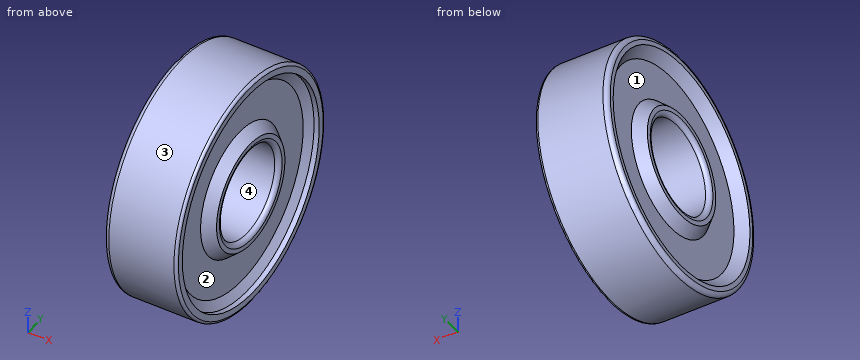
```python
from build123d import *


with BuildPart() as part:
    # Эскиз1 → Повернуть1 (revolve)
    with BuildSketch(Plane.XY):
        with BuildLine():
            Line((-3.5, 13), (3.7, 13))
            ThreePointArc((3.7, 13), (3.912132034, 12.912132034), (4, 12.7))
            Line((4, 12.7), (4, 12))
            Line((4, 12), (3.434493126, 12))
            Line((3.434493126, 12), (2.857142857, 11))
            Line((2.857142857, 11), (2.857142857, 7))
            Line((2.857142857, 7), (4, 6))
            Line((4, 6), (4, 5.5))
            ThreePointArc((4, 5.5), (3.853553391, 5.146446609), (3.5, 5))
            Line((3.5, 5), (-3.5, 5))
            ThreePointArc((-3.5, 5), (-3.853553391, 5.146446609), (-4, 5.5))
            Line((-4, 5.5), (-4, 6))
            Line((-4, 6), (-2.857142857, 7))
            Line((-2.857142857, 7), (-2.857142857, 11))
            Line((-2.857142857, 11), (-4, 12))
            Line((-4, 12), (-4, 12.5))
            ThreePointArc((-4, 12.5), (-3.853553391, 12.853553391), (-3.5, 13))
        make_face()
    revolve(axis=Axis((-1000, 0, 0), (1, 0, 0)))


solid = part.part
```
The listing builds one solid part. Answer for the finished solid, in the listing's coordinates (mm). Face numbers are marked on the shaded views. A direction names the side the tool comes from. Give positions to 0.01 mm unless a question says otherwise; leave off trailing zeros. Order: outer loops, then holes, each group sorted by start corner. A loop starts at its lowest first (then second) coordinate and runs counter-clockwise, first axis right, second up. Notation, with made-up numbers: (-31.5, 63.25) - (21.5, 63.25) arc R34 cw to (21.5, 99.25) - close; hole circle Ø10 at (-32, -14.75). An arc over 180 degrees is marked (long way). Answer in a Markdown table with one row per item. Add a question column.
Q1. For a pull along Z with two mould halves and no side action, classify the marked faces 3 and 4 as released by +Z, released by -Z, zero draft, split by the parting line, or undercut.
Q2. The part is cut by section C-C (x = -1.5). Determine the outline of the cut face in (y, z).
Q3. Which of the six approach directions +Z, -Z, +X, -X, +Y, -Y give full straight-line access (tool end or side, diameter ignored) to the marked faces 1 and 2?
Q4. Given P1, Ø1, axis at y = 1.5, z = 3, coming from the -X side; P2, Ø4, axis at x = 2, y = -9.5, coming from the -Z side; P3, Ø3, axis at x = 0, y = 9, coming from the +Z side, each flat-ended and moving along its own axis, determine where each tip first touches the part or whether it passes through.
Q5. Find the intervals of material crossed by line 1 along Z through (x, y) = (1, 0); line 2 along Z through (x, y) = (3.6, 0); line 3 along Z through (x, y) = (3.85, 0), in increasing order. Write a range as [from, to].
Determined:
| question | item | result |
|---|---|---|
| 1 | face 3 | split by the parting line |
| 1 | face 4 | undercut |
| 2 | outline | circle Ø26 at (0, 0); hole circle Ø10 at (0, 0) |
| 3 | face 1 | -X |
| 3 | face 2 | +X |
| 4 | P1 | passes through |
| 4 | P2 | stops at z = -10.62 |
| 4 | P3 | stops at z = 10.62 |
| 5 | line 1 | z = [-13, -5], [5, 13] |
| 5 | line 2 | z = [-13, -12], [-6.35, -5.01], [5.01, 6.35], [12, 13] |
| 5 | line 3 | z = [-12.96, -12], [-6.13, -5.14], [5.14, 6.13], [12, 12.96] |
